The listing builds one solid part. Answer for the finished solid, in the listing's coordinates (mm). A direction names the side the tool comes from. Coordinates: 2 decimals unless noted, no trailing zeros. Order: outer loops, then holes, each group sorted by start corner. A loop starts at its lowest first (then second) coordinate and runs counter-clockwise, first axis right, second up.
```python
from build123d import *

# Parameters (mm, degrees)
F1_DEPTH = 22.225
F2_W     = 4.7625
F2_H     = 4.7625
F3_DEPTH = 38.101
F4_R     = 1.5875


with BuildPart() as f1:
    # F0 (on Front) → F1 (new body, symmetric)
    with BuildSketch(Plane.XZ):
        Polygon((-31.75, -19.05), (31.75, -19.05), (31.75, 19.05), (1.5875, 19.05), (1.5875, 12.7), (-11.1125, 12.7), (-11.1125, 19.05), (-31.75, 19.05), align=None)
    extrude(amount=F1_DEPTH, both=True)

    # F2 (on face) → F3 (cut, through all)
    with BuildSketch(Plane.XY.offset(19.05)):
        with BuildLine():
            ThreePointArc((-26.9875, -12.7), (-25.592596, -16.067596), (-22.225, -17.4625))
            Line((-22.225, -17.4625), (-22.225, -12.7))
            Line((-22.225, -12.7), (-26.9875, -12.7))
        make_face()
        with BuildLine():
            Line((-22.225, -12.7), (-22.225, -17.4625))
            ThreePointArc((-22.225, -17.4625), (-18.857404, -16.067596), (-17.4625, -12.7))
            Line((-17.4625, -12.7), (-22.225, -12.7))
        make_face()
        with BuildLine():
            Line((-26.9875, -12.7), (-22.225, -12.7))
            Line((-22.225, -12.7), (-22.225, -7.9375))
            ThreePointArc((-22.225, -7.9375), (-25.592596, -9.332404), (-26.9875, -12.7))
        make_face()
        with BuildLine():
            Line((-22.225, -7.9375), (-22.225, -12.7))
            Line((-22.225, -12.7), (-17.4625, -12.7))
            ThreePointArc((-17.4625, -12.7), (-18.857404, -9.332404), (-22.225, -7.9375))
        make_face()
        with Locations((24.60625, 15.08125)):
            Rectangle(F2_W, F2_H)
        with Locations((19.84375, 15.08125)):
            Rectangle(F2_W, F2_H)
        with Locations((24.60625, 10.31875)):
            Rectangle(F2_W, F2_H)
        with Locations((19.84375, 10.31875)):
            Rectangle(F2_W, F2_H)
    extrude(amount=-F3_DEPTH, mode=Mode.SUBTRACT)

    # F4
    f4_edges = [f1.edges().sort_by_distance(p)[0] for p in [
        (17.4625, 17.4625, 0),
        (17.4625, 7.9375, 0),
        (26.9875, 7.9375, 0),
        (26.9875, 17.4625, 0),
    ]]
    fillet(f4_edges, radius=F4_R)


solid = f1.part
```
1) The mould has two halves that part along Y. Classify faces 1 (the cylindrical face through (26.51, 17.01, -0.27)), 2 (the flat face through (0, -22.225, 0)), 3 (the flat face through (-21, 0, 19.05)): released by +Y, released by -Y, zero draft, split by the parting line, or undercut.
2) A cutting plane is placed at A-A, the plane z = 15.5. Count the separate pieces of the cut face and the enclosed holes in it, plus the area to 3 significant figures.
3) This flat-tipped pin is pushed along its axis until it touches: P1, Ø10, axis at x = -4, y = -6.5, coming from the +Z side. Where does it stop, or does it pass through?
4) A cutting plane is placed at B-B, the plane y = -14. Write down the section's boundary in (x, z).
5) For faces 4 (the flat face through (-5, 0, 12.7)), 5 (the flat face through (22, 7.938, 0)), 6 (the flat face through (17, 0, 19.05)), determine the directions among +Z, -Z, +X, -X, +Y, -Y from which every point of the face is accessible in a straight line to the end or side of a thin tool.
6) A cutting plane is placed at C-C, the plane y = -4.5. Write down the section's boundary in (x, z), plus the area to 3 significant figures.
7) Straight lines are drawn through the part: probe 1 along X at (y, z) = (13.5, 17.5); probe 2 along X at (y, z) = (12.5, 7.5); probe 3 along Y at (x, z) = (-22.5, -12) (3 decimals). For each, find the intervals that lie inside material, in ascending order.
Working result:
1. face 1: undercut
1. face 2: released by -Y
1. face 3: zero draft
2. separate pieces: 2
2. enclosed holes: 2
2. area: 2,100 mm2
3. P1: stops at z = 12.7
4. outline: (-31.75, -19.05) - (-26.81, -19.05) - (-26.81, 19.05) - (-31.75, 19.05) - close; (-17.64, -19.05) - (31.75, -19.05) - (31.75, 19.05) - (1.59, 19.05) - (1.59, 12.7) - (-11.11, 12.7) - (-11.11, 19.05) - (-17.64, 19.05) - close
5. face 4: +Z, +Y, -Y
5. face 5: +Z, -Z
5. face 6: +Z, +X, -X, +Y, -Y
6. outline: (-31.75, -19.05) - (31.75, -19.05) - (31.75, 19.05) - (1.59, 19.05) - (1.59, 12.7) - (-11.11, 12.7) - (-11.11, 19.05) - (-31.75, 19.05) - close
6. area: 2,340 mm2
7. probe 1: x = -31.75 to -11.11, 1.59 to 17.46, 26.99 to 31.75
7. probe 2: x = -31.75 to 17.46, 26.99 to 31.75
7. probe 3: y = -22.225 to -17.455, -7.945 to 22.225
